from build123d import *

# Parameters (mm, degrees)
BOSS_EXTRUDE1_DEPTH = 76.2
SKETCH3_W           = 8.774879522
SKETCH3_H           = 8.636
CUT_EXTRUDE1_DEPTH  = 33.02
SKETCH5_W           = 1.27
SKETCH5_H           = 2.54
CUT_EXTRUDE2_DEPTH  = 1.5
BOSS_EXTRUDE2_DEPTH = 76.2
SKETCH7_R           = 1.55
CUT_EXTRUDE3_DEPTH  = 3.2766
SKETCH9_R           = 1.55
CUT_EXTRUDE4_DEPTH  = 1.5


with BuildPart() as part:
    # Sketch1 → Boss-Extrude1 (new body)
    with BuildSketch(Plane.XY):
        Polygon((3.772933373, -7.404439667), (0.641286927, -10.681039667), (36.201286927, -10.681039667), (36.201286927, -7.404439667), align=None)
        Polygon((57.914204847, 51.413822136), (58.998579611, 50.377419043), (0.641286927, -10.681039667), (-12.283449407, -10.681039667), (-1.084374764, 1.036403093), (0, 0), (-8.774879522, -9.181039667), (0, -9.181039667), align=None)
    extrude(amount=BOSS_EXTRUDE1_DEPTH)

    # Sketch3 → Cut-Extrude1 (cut, symmetric)
    with BuildSketch(Plane(origin=(0, -9.181039667, 0), x_dir=(1, 0, 0), z_dir=(0, 1, 0))):
        with Locations((-4.387439761, -42.418)):
            Rectangle(SKETCH3_W, SKETCH3_H)
        with Locations((-4.387439761, -33.782)):
            Rectangle(SKETCH3_W, SKETCH3_H)
    extrude(amount=CUT_EXTRUDE1_DEPTH, both=True, mode=Mode.SUBTRACT)

    # Sketch5 → Cut-Extrude2 (cut)
    with BuildSketch(Plane(origin=(4.585824688, -4.382952324, 0), x_dir=(0, 0, 1), z_dir=(-0.722916509, 0.690935395, 0))):
        with Locations((3.175, 22.572874853)):
            Rectangle(SKETCH5_W, SKETCH5_H)
        with Locations((3.175, 35.272874853)):
            Rectangle(SKETCH5_W, SKETCH5_H)
        with Locations((3.175, 47.972874853)):
            Rectangle(SKETCH5_W, SKETCH5_H)
        with Locations((73.025, 22.572874853)):
            Rectangle(SKETCH5_W, SKETCH5_H)
        with Locations((73.025, 35.272874853)):
            Rectangle(SKETCH5_W, SKETCH5_H)
        with Locations((73.025, 47.972874853)):
            Rectangle(SKETCH5_W, SKETCH5_H)
    extrude(amount=-CUT_EXTRUDE2_DEPTH, mode=Mode.SUBTRACT)

    # Sketch6 → Boss-Extrude2 (add)
    with BuildSketch(Plane.XY.offset(76.2)):
        Polygon((23.628168528, -7.404439667), (23.628168528, 13.36982864), (27.885054397, 17.823751673), (28.455712225, -7.404439667), align=None)
    extrude(amount=-BOSS_EXTRUDE2_DEPTH)

    # Sketch7 → Cut-Extrude3 (cut)
    with BuildSketch(Plane(origin=(0, -7.404439667, 0), x_dir=(1, 0, 0), z_dir=(0, 1, 0))):
        with Locations((32.265712225, -72.39)):
            Circle(SKETCH7_R)
        with Locations((32.265712225, -3.81)):
            Circle(SKETCH7_R)
        with Locations((32.265712225, -38.1)):
            Circle(SKETCH7_R)
    extrude(amount=-CUT_EXTRUDE3_DEPTH, mode=Mode.SUBTRACT)

    # Sketch9 → Cut-Extrude4 (cut)
    with BuildSketch(Plane(origin=(0, -9.181039667, 0), x_dir=(1, 0, 0), z_dir=(0, 1, 0))):
        with Locations((-4.329879522, -61.468)):
            Circle(SKETCH9_R)
        with Locations((-4.329879522, -14.732)):
            Circle(SKETCH9_R)
    extrude(amount=-CUT_EXTRUDE4_DEPTH, mode=Mode.SUBTRACT)


solid = part.part
The model under review builds one solid part; all positions refer to its coordinate system, in mm. A direction names the side the tool comes from. Give positions to 0.01 mm unless a question says otherwise; leave off trailing zeros. Order: outer loops, then holes, each group sorted by start corner. A loop starts at its lowest first (then second) coordinate and runs counter-clockwise, first axis right, second up. Notation, with made-up numbers: M 40.25,87.25 L 55.25,87.25 A29 cw 55.25,123.25 Z; hole C 60.25,-17 d10. An arc over 180 degrees is marked long. One line per question, with ' | ' between items. Start each with the question number.
1) Consider section B-B, the plane z = 38.1. Give the boundary of the cut face in (x, y), then the cut area to 3 significant figures.
2) Clearance check with flat-ended pins moving along their axes: P1, Ø1.2, axis at y = -10, z = 38, coming from the -X side; P2, Ø6, axis at x = 8, z = 32, coming from the +Y side; P3, Ø6, axis at y = 32, z = 23, coming from the +X side; P4, Ø10, axis at x = 37.5, y = 42, coming from the -Z side. State where each tip first meets the part, or that it passes through.
3) For faces 5 (the face through (38, 30, 3.81)), 6 (the face through (-4.3, -4.5, 14.5)), 7 (the face through (43.66, 34.33, 37.57)), 8 (the face through (28.55, 20.69, 37.57)), 9 (the face through (31.036, -9.02, 73.333)), list the 3-axis set-ups (+Z, -Z, +X, -X, +Y, -Y) from which the entire face can be reached by the end or side of a thin tool; tool diameter is ignored.
4) Consider section A-A, the plane z = 10.5. Give the boundary of the cut face in (x, y).
5) Mouldability with a two-part tool opening along Y and no side actions: class faces 1 (the face through (-9.25, -7.51, 37.57)), 2 (the face through (30.717, -9.02, 3.742)), 3 (the face through (23.628, 3, 39)), 4 (the face through (-6, -9.181, 61)) as pulls with the +Y half, pulls with the -Y half, needs draft (parallel to the pull), parting line crosses it, or undercut.
6) Consider section C-C, the plane y = -5.5. Give the boundary of the cut face in (x, z).
7) Consider section D-D, the plane x = 6.5. Give the boundary of the cut face in (y, z).
8) Wall thickness on L1, parallel to X at y = -8.55, z = 72.39; L2, parallel to X at y = -9, z = 38; L3, parallel to Y at x = 30, z = 39.5: over which ranges is each line inside the solid? List them lowest first. Write a range as from..to.
Found:
1) outline: M -12.28,-10.68 L -8.77,-10.68 L -8.77,-7.01 Z; M 0,-10.68 L 30.72,-10.68 L 30.72,-7.4 L 28.46,-7.4 L 27.89,17.82 L 59,50.38 L 57.91,51.41 L 0,-9.18 Z; M 33.82,-10.68 L 36.2,-10.68 L 36.2,-7.4 L 33.82,-7.4 Z; hole M 3.77,-7.4 L 23.63,-7.4 L 23.63,13.37 Z | area: 339 mm²
2) P1: stops at x = -12.21 | P2: stops at y = 2.33 | P3: stops at x = 44.3 | P4: passes through
3) face 5: none | face 6: +Z, -Z | face 7: +Z, -Z, +X | face 8: +Z, -Z, +Y | face 9: -Y
4) outline: M -12.28,-10.68 L 36.2,-10.68 L 36.2,-7.4 L 28.46,-7.4 L 27.89,17.82 L 59,50.38 L 57.91,51.41 L 0,-9.18 L -8.77,-9.18 L 0,0 L -1.08,1.04 Z; hole M 3.77,-7.4 L 23.63,-7.4 L 23.63,13.37 Z
5) face 1: pulls with the +Y half | face 2: needs draft | face 3: undercut | face 4: undercut
6) outline: M -7.33,0 L -5.26,0 L -5.26,29.46 L -7.33,29.46 Z; M -7.33,46.74 L -5.26,46.74 L -5.26,76.2 L -7.33,76.2 Z; M 3.52,0 L 5.59,0 L 5.59,76.2 L 3.52,76.2 Z; M 23.63,0 L 28.41,0 L 28.41,76.2 L 23.63,76.2 Z
7) outline: M -10.68,0 L -7.4,0 L -7.4,76.2 L -10.68,76.2 Z; M -4.55,0 L -2.38,0 L -2.38,76.2 L -4.55,76.2 Z
8) L1: x = -10.25..-8.17, 0.6..30.72, 33.82..36.2 | L2: x = -10.68..-8.77, 0.17..30.72, 33.81..36.2 | L3: y = -10.68..-7.4, 20.04..22.21
